Model file for the job. Use its own axes, mm. A direction names the side the tool comes from. Give positions to 0.01 mm unless a question says otherwise; leave off trailing zeros. Write each loop counter-clockwise with the first axis right and the second up, starting at its lowest first coordinate (ties: lowest second). Pieces come first, ordered by that corner, then holes. Notation, with made-up numbers: (8, 41) - (51, 41) arc R8 cw to (51, 53) - close; hole circle Ø7 at (53.25, 84.25). An arc over 180 degrees is marked (long way). Use a Markdown table: item, result. Add a question column.
```python
from build123d import *

# Parameters (mm, degrees)
F0_W     = 17
F0_H     = 7.35
F1_DEPTH = 70
F3_DEPTH = 50


with BuildPart() as f1:
    # F0 (on Front) → F1 (new body)
    with BuildSketch(Plane.XZ):
        Rectangle(F0_W, F0_H)
    extrude(amount=-F1_DEPTH)

    # F2 (on face) → F3 (cut)
    with BuildSketch(Plane.XZ):
        Polygon((-3.425, -0.825), (-3.425, -3.675), (3.425, -3.675), (3.425, -0.825), (5.93029, -0.825), (5.93029, 1.575), (-5.93029, 1.575), (-5.93029, -0.825), align=None)
    extrude(amount=-F3_DEPTH, mode=Mode.SUBTRACT)


solid = f1.part
```
(1) Probe probe 1 along X at (y, z) = (16, 1); probe 2 along X at (y, z) = (18, -2.5) (3 decimals); probe 3 along Z at (x, y) = (3.5, 19) (3 decimals). List the from-to ranges inside material, lowest first. Write a range as [from, to].
(2) Two-plate mould, pull along Z, no slides. Class faces 4 (the flat face through (0, 50, 0)), 5 (the flat face through (4, 35, -3.675)), 6 (the flat face through (-8.5, 35, 0)), 7 (the flat face through (5.93, 25, 0)): +Z half, -Z half, draft (parallel to the pull), parting line (faces both ways), or undercut.
(3) Which spindle directions (+Z, -Z, +X, -X, +Y, -Y) get a long thin tool onto all of the face, cutting with end or side? Do faces 1 (the flat face through (3.425, 25, -2)), 2 (the flat face through (-5.93, 25, 0)), 3 (the flat face through (0, 0, 2)). Say none if no direction does.
(4) Flat gauge pin, fed straight in: pin 1 (1.5 mm diameter, centred on x = 1.5, z = -2, fed in from -Y). Where does the tip first touch, or does it go through?
(5) Band-saw the part on A-A (x = -1.5). Write the cut outline in (y, z) (3 decimals).
(6) Band-saw the part on C-C (z = -1.5). Write the cut outline in (x, y) (3 decimals), then the cut area to 4 significant figures.
(7) Band-saw the part on B-B (y = 9.5). Write the cut outline in (x, z) (3 decimals), then the cut area to 3 significant figures.
Model answer:
| question | item | result |
|---|---|---|
| 1 | probe 1 | x = [-8.5, -5.93], [5.93, 8.5] |
| 1 | probe 2 | x = [-8.5, -3.425], [3.425, 8.5] |
| 1 | probe 3 | z = [-3.675, -0.825], [1.575, 3.675] |
| 2 | face 4 | undercut |
| 2 | face 5 | -Z half |
| 2 | face 6 | draft |
| 2 | face 7 | undercut |
| 3 | face 1 | -Z, -Y |
| 3 | face 2 | -Y |
| 3 | face 3 | +Z, -Z, +X, -X, -Y |
| 4 | pin 1 | stops at y = 50 |
| 5 | outline | (0, 1.575) - (50, 1.575) - (50, -3.675) - (70, -3.675) - (70, 3.675) - (0, 3.675) - close |
| 6 | outline | (-8.5, 0) - (-3.425, 0) - (-3.425, 50) - (3.425, 50) - (3.425, 0) - (8.5, 0) - (8.5, 70) - (-8.5, 70) - close |
| 6 | area | 847.5 mm^2 |
| 7 | outline | (-8.5, -3.675) - (-3.425, -3.675) - (-3.425, -0.825) - (-5.93, -0.825) - (-5.93, 1.575) - (5.93, 1.575) - (5.93, -0.825) - (3.425, -0.825) - (3.425, -3.675) - (8.5, -3.675) - (8.5, 3.675) - (-8.5, 3.675) - close |
| 7 | area | 77.0 mm^2 |
